Geometry: final body of the model. Coordinates: model frame, mm. A direction names the side the tool comes from. Round coordinates to 2 decimals unless told otherwise and drop trailing zeros. Loops run counter-clockwise (first coordinate to the right, second up) from the corner with the lowest first, then second, coordinate; pieces in that order, holes last. Notation, with made-up numbers: (50.5, -23.5) - (81.5, -23.5) arc R22 cw to (81.5, -12.5) - close; hole circle Ø2 at (2, -38.75). An arc over 180 degrees is marked (long way). Answer as a JSON object with one key per item and string values. Group by question number.
Item 1: Section A-A (y = 172.5). Return the cut outline in (x, z).
Item 2: Draft query along Y for faces 3 (the face through (252.91, -219.4, 1.48)), 4 (the face through (269.61, -243.27, 1.48)), 5 (the face through (250, 33, 3)). Return one class per face: released by +Y, released by -Y, zero draft, split by the parting line, or undercut.
Item 3: Reachability of faces 1 (the face through (250, 33, 0)), 2 (the face through (247.083, -28.989, 1.479)) from +Z, -Z, +X, -X, +Y, -Y: full face, straight path, thin tool, end or side. Return the list, or none.
Item 4: First-contact query: pin 1 (1.5 mm diameter, centred on x = 271, z = 1.5, fed in from -Y); pin 2 (1 mm diameter, centred on y = -79.5, z = 2.5, fed in from -X); pin 3 (1.2 mm diameter, centred on y = -240, z = 2, fed in from +X). Flat tips, straight axial feed; report the tip coordinate or a pass-through.
Item 5: Section B-B (z = 2.1). Count the separate pieces of the cut face and the enclosed holes in it, plus the area to 3 significant figures.
Item 6: Line query: line 1 (Y direction, x = 222.5, z = 0.55); line 2 (Y direction, x = 222, z = 0.75); line 3 (X direction, y = 41.5, z = 2). Output: solid intervals per line, ascending.
```python
from build123d import *

# Parameters (mm, degrees)
SKETCH_1_R      = 10
SKETCH_1_R_2    = 2
SKETCH_1_R_3    = 5.5
EXTRUDE_1_DEPTH = 3


with BuildPart() as part:
    # 草图1 → 凸台-拉伸1 (new body)
    with BuildSketch(Plane.XY):
        with BuildLine():
            Line((224.953360513, -85.216557036), (224.953360513, -86.716557036))
            Line((224.953360513, -86.716557036), (227.553360513, -86.716557036))
            Line((227.553360513, -86.716557036), (227.553360513, -85.216557036))
            Line((227.553360513, -85.216557036), (230.553360513, -85.216557036))
            Line((230.553360513, -85.216557036), (230.553360513, -82.216557036))
            Line((230.553360513, -82.216557036), (227.553360513, -82.216557036))
            Line((227.553360513, -82.216557036), (227.553360513, -80.716557036))
            Line((227.553360513, -80.716557036), (224.953360513, -80.716557036))
            Line((224.953360513, -80.716557036), (224.953360513, -82.216557036))
            Line((224.953360513, -82.216557036), (222.453360513, -82.216557036))
            Line((222.453360513, -82.216557036), (222.453360513, 78.373187283))
            Line((222.453360513, 78.373187283), (219.453360513, 78.373187283))
            Line((219.453360513, 78.373187283), (219.453360513, 82.373187283))
            Line((219.453360513, 82.373187283), (219.453360513, 86.373187283))
            Line((219.453360513, 86.373187283), (222.453360513, 86.373187283))
            Line((222.453360513, 86.373187283), (222.453360513, 246.962931603))
            Line((222.453360513, 246.962931603), (224.953360513, 246.962931603))
            Line((224.953360513, 246.962931603), (224.953360513, 245.462931603))
            Line((224.953360513, 245.462931603), (227.553360513, 245.462931603))
            Line((227.553360513, 245.462931603), (227.553360513, 246.962931603))
            Line((227.553360513, 246.962931603), (230.553360513, 246.962931603))
            Line((230.553360513, 246.962931603), (230.553360513, 249.962931603))
            Line((230.553360513, 249.962931603), (227.553360513, 249.962931603))
            Line((227.553360513, 249.962931603), (227.553360513, 251.462931603))
            Line((227.553360513, 251.462931603), (224.953360513, 251.462931603))
            Line((224.953360513, 251.462931603), (224.953360513, 249.962931603))
            Line((224.953360513, 249.962931603), (222.453360513, 249.962931603))
            Line((222.453360513, 249.962931603), (222.453360513, 275.962931603))
            Line((222.453360513, 275.962931603), (222.453360513, 301.962931603))
            Line((222.453360513, 301.962931603), (224.953360513, 301.962931603))
            Line((224.953360513, 301.962931603), (224.953360513, 300.462931603))
            Line((224.953360513, 300.462931603), (227.553360513, 300.462931603))
            Line((227.553360513, 300.462931603), (227.553360513, 301.962931603))
            Line((227.553360513, 301.962931603), (230.553360513, 301.962931603))
            Line((230.553360513, 301.962931603), (230.553360513, 304.962931603))
            Line((230.553360513, 304.962931603), (227.553360513, 304.962931603))
            Line((227.553360513, 304.962931603), (227.553360513, 306.462931603))
            Line((227.553360513, 306.462931603), (224.953360513, 306.462931603))
            Line((224.953360513, 306.462931603), (224.953360513, 304.962931603))
            Line((224.953360513, 304.962931603), (222.453360513, 304.962931603))
            Line((222.453360513, 304.962931603), (222.453360513, 309.962931603))
            Line((222.453360513, 309.962931603), (277.453360513, 309.962931603))
            Line((277.453360513, 309.962931603), (277.453360513, 304.962931603))
            Line((277.453360513, 304.962931603), (274.953360513, 304.962931603))
            Line((274.953360513, 304.962931603), (274.953360513, 306.462931603))
            Line((274.953360513, 306.462931603), (272.353360513, 306.462931603))
            Line((272.353360513, 306.462931603), (272.353360513, 304.962931603))
            Line((272.353360513, 304.962931603), (269.353360513, 304.962931603))
            Line((269.353360513, 304.962931603), (269.353360513, 301.962931603))
            Line((269.353360513, 301.962931603), (272.353360513, 301.962931603))
            Line((272.353360513, 301.962931603), (272.353360513, 300.462931603))
            Line((272.353360513, 300.462931603), (274.953360513, 300.462931603))
            Line((274.953360513, 300.462931603), (274.953360513, 301.962931603))
            Line((274.953360513, 301.962931603), (277.453360513, 301.962931603))
            Line((277.453360513, 301.962931603), (277.453360513, 249.962931603))
            Line((277.453360513, 249.962931603), (274.953360513, 249.962931603))
            Line((274.953360513, 249.962931603), (274.953360513, 251.462931603))
            Line((274.953360513, 251.462931603), (272.353360513, 251.462931603))
            Line((272.353360513, 251.462931603), (272.353360513, 249.962931603))
            Line((272.353360513, 249.962931603), (269.353360513, 249.962931603))
            Line((269.353360513, 249.962931603), (269.353360513, 246.962931603))
            Line((269.353360513, 246.962931603), (272.353360513, 246.962931603))
            Line((272.353360513, 246.962931603), (272.353360513, 245.462931603))
            Line((272.353360513, 245.462931603), (274.953360513, 245.462931603))
            Line((274.953360513, 245.462931603), (274.953360513, 246.962931603))
            Line((274.953360513, 246.962931603), (277.453360513, 246.962931603))
            Line((277.453360513, 246.962931603), (277.453360513, 196.052675922))
            Line((277.453360513, 196.052675922), (280.453360513, 196.052675922))
            Line((280.453360513, 196.052675922), (280.453360513, 192.052675922))
            Line((280.453360513, 192.052675922), (280.453360513, 188.052675922))
            Line((280.453360513, 188.052675922), (277.453360513, 188.052675922))
            Line((277.453360513, 188.052675922), (277.453360513, 137.142420241))
            Line((277.453360513, 137.142420241), (274.953360513, 137.142420241))
            Line((274.953360513, 137.142420241), (274.953360513, 138.642420241))
            Line((274.953360513, 138.642420241), (272.353360513, 138.642420241))
            Line((272.353360513, 138.642420241), (272.353360513, 137.142420241))
            Line((272.353360513, 137.142420241), (269.353360513, 137.142420241))
            Line((269.353360513, 137.142420241), (269.353360513, 134.142420241))
            Line((269.353360513, 134.142420241), (272.353360513, 134.142420241))
            Line((272.353360513, 134.142420241), (272.353360513, 132.642420241))
            Line((272.353360513, 132.642420241), (274.953360513, 132.642420241))
            Line((274.953360513, 132.642420241), (274.953360513, 134.142420241))
            Line((274.953360513, 134.142420241), (277.453360513, 134.142420241))
            Line((277.453360513, 134.142420241), (277.453360513, -26.447324078))
            Line((277.453360513, -26.447324078), (280.453360513, -26.447324078))
            Line((280.453360513, -26.447324078), (280.453360513, -30.447324078))
            Line((280.453360513, -30.447324078), (280.453360513, -34.447324078))
            Line((280.453360513, -34.447324078), (277.453360513, -34.447324078))
            Line((277.453360513, -34.447324078), (277.453360513, -195.037068397))
            Line((277.453360513, -195.037068397), (274.953360513, -195.037068397))
            Line((274.953360513, -195.037068397), (274.953360513, -193.537068397))
            Line((274.953360513, -193.537068397), (272.353360513, -193.537068397))
            Line((272.353360513, -193.537068397), (272.353360513, -195.037068397))
            Line((272.353360513, -195.037068397), (269.353360513, -195.037068397))
            Line((269.353360513, -195.037068397), (269.353360513, -198.037068397))
            Line((269.353360513, -198.037068397), (272.353360513, -198.037068397))
            Line((272.353360513, -198.037068397), (272.353360513, -199.537068397))
            Line((272.353360513, -199.537068397), (274.953360513, -199.537068397))
            Line((274.953360513, -199.537068397), (274.953360513, -198.037068397))
            Line((274.953360513, -198.037068397), (277.453360513, -198.037068397))
            Line((277.453360513, -198.037068397), (277.453360513, -224.037068397))
            ThreePointArc((277.453360513, -224.037068397), (269.398796996, -243.48250488), (249.953360513, -251.537068397))
            Line((249.953360513, -251.537068397), (222.453360513, -251.537068397))
            Line((222.453360513, -251.537068397), (222.453360513, -239.287068397))
            Line((222.453360513, -239.287068397), (224.953360513, -239.287068397))
            Line((224.953360513, -239.287068397), (224.953360513, -240.787068397))
            Line((224.953360513, -240.787068397), (227.553360513, -240.787068397))
            Line((227.553360513, -240.787068397), (227.553360513, -239.287068397))
            Line((227.553360513, -239.287068397), (230.553360513, -239.287068397))
            Line((230.553360513, -239.287068397), (230.553360513, -236.287068397))
            Line((230.553360513, -236.287068397), (227.553360513, -236.287068397))
            Line((227.553360513, -236.287068397), (227.553360513, -234.787068397))
            Line((227.553360513, -234.787068397), (224.953360513, -234.787068397))
            Line((224.953360513, -234.787068397), (224.953360513, -236.287068397))
            Line((224.953360513, -236.287068397), (222.453360513, -236.287068397))
            Line((222.453360513, -236.287068397), (222.453360513, -224.037068397))
            Line((222.453360513, -224.037068397), (222.453360513, -198.037068397))
            Line((222.453360513, -198.037068397), (224.953360513, -198.037068397))
            Line((224.953360513, -198.037068397), (224.953360513, -199.537068397))
            Line((224.953360513, -199.537068397), (227.553360513, -199.537068397))
            Line((227.553360513, -199.537068397), (227.553360513, -198.037068397))
            Line((227.553360513, -198.037068397), (230.553360513, -198.037068397))
            Line((230.553360513, -198.037068397), (230.553360513, -195.037068397))
            Line((230.553360513, -195.037068397), (227.553360513, -195.037068397))
            Line((227.553360513, -195.037068397), (227.553360513, -193.537068397))
            Line((227.553360513, -193.537068397), (224.953360513, -193.537068397))
            Line((224.953360513, -193.537068397), (224.953360513, -195.037068397))
            Line((224.953360513, -195.037068397), (222.453360513, -195.037068397))
            Line((222.453360513, -195.037068397), (222.453360513, -144.126812717))
            Line((222.453360513, -144.126812717), (219.453360513, -144.126812717))
            Line((219.453360513, -144.126812717), (219.453360513, -140.126812717))
            Line((219.453360513, -140.126812717), (219.453360513, -136.126812717))
            Line((219.453360513, -136.126812717), (222.453360513, -136.126812717))
            Line((222.453360513, -136.126812717), (222.453360513, -85.216557036))
            Line((222.453360513, -85.216557036), (224.953360513, -85.216557036))
        make_face()
        with Locations((249.953360513, 275.962931603)):
            Circle(SKETCH_1_R, mode=Mode.SUBTRACT)
        with Locations((230.953360513, 275.962931603)):
            Circle(SKETCH_1_R_2, mode=Mode.SUBTRACT)
        with Locations((236.518331671, 289.397960445)):
            Circle(SKETCH_1_R_2, mode=Mode.SUBTRACT)
        with Locations((249.953360513, 294.962931603)):
            Circle(SKETCH_1_R_2, mode=Mode.SUBTRACT)
        with Locations((263.388389356, 289.397960445)):
            Circle(SKETCH_1_R_2, mode=Mode.SUBTRACT)
        with Locations((268.953360513, 275.962931603)):
            Circle(SKETCH_1_R_2, mode=Mode.SUBTRACT)
        with Locations((263.388389356, 262.52790276)):
            Circle(SKETCH_1_R_2, mode=Mode.SUBTRACT)
        with Locations((249.953360513, 256.962931603)):
            Circle(SKETCH_1_R_2, mode=Mode.SUBTRACT)
        with Locations((236.518331671, 262.52790276)):
            Circle(SKETCH_1_R_2, mode=Mode.SUBTRACT)
        with Locations((249.953360513, -224.037068397)):
            Circle(SKETCH_1_R_3, mode=Mode.SUBTRACT)
        with BuildLine():
            Line((233.453360513, 232.962931603), (265.776162867, 232.962931603))
            ThreePointArc((265.776162867, 232.962931603), (268.007619579, 231.968075224), (268.759090329, 229.643332232))
            Line((268.759090329, 229.643332232), (236.436287975, -72.036156407))
            ThreePointArc((236.436287975, -72.036156407), (233.293332993, -74.712285861), (230.453360513, -71.716557036))
            Line((230.453360513, -71.716557036), (230.453360513, 229.962931603))
            ThreePointArc((230.453360513, 229.962931603), (231.33204017, 232.084251946), (233.453360513, 232.962931603))
        make_face(mode=Mode.SUBTRACT)
        with BuildLine():
            Line((269.453360513, 123.642420241), (269.453360513, -178.037068397))
            ThreePointArc((269.453360513, -178.037068397), (268.574680857, -180.158388741), (266.453360513, -181.037068397))
            Line((266.453360513, -181.037068397), (234.130558159, -181.037068397))
            ThreePointArc((234.130558159, -181.037068397), (231.899101447, -180.042212019), (231.147630697, -177.717469026))
            Line((231.147630697, -177.717469026), (263.470433052, 123.962019612))
            ThreePointArc((263.470433052, 123.962019612), (266.613388034, 126.638149066), (269.453360513, 123.642420241))
        make_face(mode=Mode.SUBTRACT)
    extrude(amount=EXTRUDE_1_DEPTH)


solid = part.part
```
Values:
{
 "1": {"outline": "(222.45, 0) - (230.45, 0) - (230.45, 3) - (222.45, 3) - close; (262.64, 0) - (277.45, 0) - (277.45, 3) - (262.64, 3) - close"},
 "2": {"face 3": "undercut", "face 4": "released by -Y", "face 5": "zero draft"},
 "3": {"face 1": "-Z, +X, -X, +Y, -Y", "face 2": "+Z, -Z"},
 "4": {"pin 1": "stops at y = -242.59", "pin 2": "stops at x = 222.45", "pin 3": "stops at x = 272.76"},
 "5": {"separate pieces": "1", "enclosed holes": "12", "area": "16,400 mm^2"},
 "6": {"line 1": "y = -251.54 to -239.29, -236.29 to -198.04, -195.04 to -85.22, -82.22 to 246.96, 249.96 to 301.96, 304.96 to 309.96", "line 2": "y = -144.13 to -136.13, 78.37 to 86.37", "line 3": "x = 222.45 to 230.45, 248.6 to 254.64, 269.45 to 277.45"}
}
